Verification items for this drawing (mm, ordinates from the low corner). A direction names the side the tool comes from. Give positions to 0.01 mm unless a question says otherwise; leave off trailing zeros. Loops run counter-clockwise (first coordinate to the right, second up) from the corner with the lowest first, then second, coordinate; pieces in that order, holes last. Notation, with made-up numbers: (11.25, -0.75) -> (27.25, -0.75) arc R27 ccw to (27.25, 25.25) -> close; hole circle Ø6 at (63.25, 17). An arc over 180 degrees is marked (long way). Answer as a JSON object with one key per item and string values.
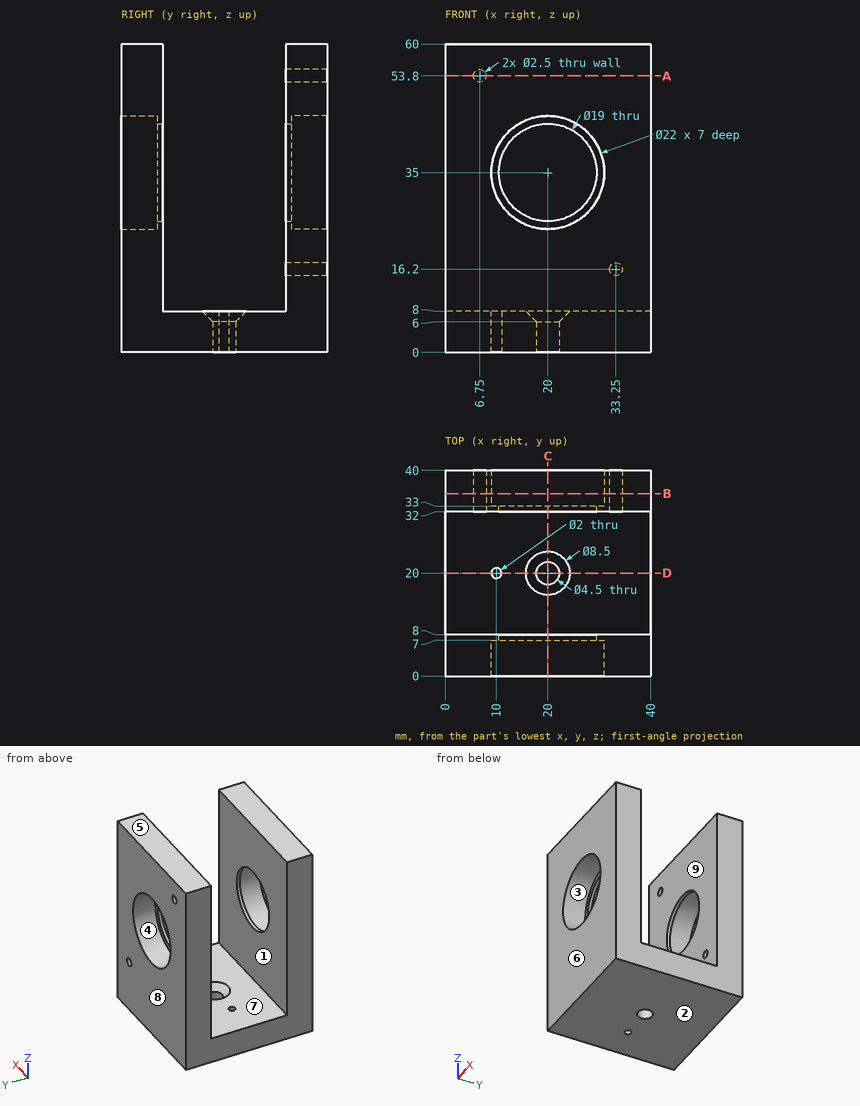
1) Draft check along Y on the marked faces 6, 7, 8 and 9. Enter one of: pulls with the +Y half, pulls with the -Y half, needs draft (parallel to the pull), parting line crosses it, or undercut.
Geometry check:
{"face 6": "pulls with the -Y half", "face 7": "undercut", "face 8": "pulls with the +Y half", "face 9": "undercut"}
2) Material ranges on line 1 along Y through (x, z) = (9, 37); line 2 along X through (y, z) = (35.25, 53.8); line 3 along X through (y, z) = (7.45, 35), recorded low to high. Write a range as from..to.
Geometry check:
{"line 1": "y = 0..8, 32..40", "line 2": "x = 0..5.5, 8..40", "line 3": "x = 0..10.5, 29.5..40"}
3) Section check A-A on z = 53.8. Record the cut outline in (x, y), plus the area to 3 significant figures.
Geometry check:
{"outline": "(0, 0) -> (40, 0) -> (40, 8) -> (0, 8) -> close; (0, 32) -> (5.5, 32) -> (5.5, 40) -> (0, 40) -> close; (8, 32) -> (40, 32) -> (40, 40) -> (8, 40) -> close", "area": "620 mm2"}
4) Tool access check on the marked faces 1, 2, 3, 4 and 5. Record the directions out of +Z, -Z, +X, -X, +Y, -Y that give a thin tool (end or side, any length) a straight path to the whole face; none if there is none.
Geometry check:
{"face 1": "+Z, +X, -X", "face 2": "-Z, +X, -X, +Y, -Y", "face 3": "-Y", "face 4": "+Y", "face 5": "+Z, +X, -X, +Y, -Y"}
5) Section check C-C on x = 20. Count the separate pieces of the cut face and the enclosed holes in it, plus the area to 3 significant figures.
Geometry check:
{"separate pieces": "4", "enclosed holes": "0", "area": "766 mm2"}
6) Section check B-B on y = 35.5. Record the cut outline in (x, z), plus the area to 3 significant figures.
Geometry check:
{"outline": "(0, 0) -> (40, 0) -> (40, 60) -> (0, 60) -> close; hole circle Ø2.5 at (6.75, 53.8); hole circle Ø22 at (20, 35); hole circle Ø2.5 at (33.25, 16.2)", "area": "2,010 mm2"}
7) Depth check by flat-ended pin: P1, Ø13, axis at x = 20, z = 35, coming from the -Y side; P2, Ø5, axis at x = 18, y = 13.5, coming from the +Z side. Enter the tip coordinate at first touch or a pass-through.
Geometry check:
{"P1": "passes through", "P2": "stops at z = 8"}
8) Section check D-D on y = 20. Record the cut outline in (x, z), plus the area to 3 significant figures.
Geometry check:
{"outline": "(0, 0) -> (9, 0) -> (9, 8) -> (0, 8) -> close; (11, 0) -> (17.75, 0) -> (17.75, 6) -> (15.75, 8) -> (11, 8) -> close; (22.25, 0) -> (40, 0) -> (40, 8) -> (24.25, 8) -> (22.25, 6) -> close", "area": "264 mm2"}
